Build history of the part. All positions in model axes, mm. A direction names the side the tool comes from. Coordinates: 2 decimals unless noted, no trailing zeros. Order: outer loops, then holes, each group sorted by start corner. A loop starts at its lowest first (then second) coordinate and runs counter-clockwise, first axis right, second up. Notation, with made-up numbers: (8.5, -10.75) - (13.5, -10.75) arc R14 ccw to (13.5, 10.25) - close; hole circle Ø2 at (-37, 20.25). An arc over 180 degrees is marked (long way). Answer as CSV lines item,"result". Start each with the question number.
from build123d import *

# Parameters (mm, degrees)
BOSS_EXTRUDE1_DEPTH = 90
SKETCH2_R           = 2
CUT_EXTRUDE1_DEPTH  = 26
BOSS_EXTRUDE2_DEPTH = 90
SKETCH4_W           = 47.922407602
SKETCH4_H           = 26.699627092
BOSS_EXTRUDE3_DEPTH = 20
SKETCH7_R           = 2.5
CUT_EXTRUDE2_DEPTH  = 66.5
SKETCH9_W           = 15
SKETCH9_H           = 8
CUT_EXTRUDE3_DEPTH  = 91
CUT_EXTRUDE4_REACH  = 62.6
SKETCH8_R           = 2.5
CUT_EXTRUDE5_DEPTH  = 67
SKETCH12_W          = 63.84660413
SKETCH12_H          = 90
BOSS_EXTRUDE4_DEPTH = 67
BOSS_EXTRUDE5_START = -3
SKETCH13_R          = 10
BOSS_EXTRUDE5_DEPTH = 31
SKETCH15_R          = 12.5
BOSS_EXTRUDE6_DEPTH = 3
SKETCH16_R          = 12.5
BOSS_EXTRUDE7_DEPTH = 3
SKETCH17_W          = 34
SKETCH17_H          = 34
CUT_EXTRUDE6_DEPTH  = 2
SKETCH18_R          = 10
CUT_EXTRUDE7_DEPTH  = 5
SKETCH19_R          = 12.5
CUT_EXTRUDE8_DEPTH  = 3


with BuildPart() as part:
    # Sketch1 → Boss-Extrude1 (new body)
    with BuildSketch(Plane.XY):
        Polygon((-283, 0), (0, 0), (0, 15), (-217.53, 15), (-217.53, 11), (-237.53, 11), (-237.53, 15), (-254.5, 15), (-254.5, 11), (-274, 11), (-274, 15), (-283, 15), align=None)
    extrude(amount=BOSS_EXTRUDE1_DEPTH)

    # Sketch2 → Cut-Extrude1 (cut)
    with BuildSketch(Plane(origin=(0, 15, 0), x_dir=(1, 0, 0), z_dir=(0, 1, 0))):
        with Locations((-246.015, -45)):
            Circle(SKETCH2_R)
    extrude(amount=-CUT_EXTRUDE1_DEPTH, mode=Mode.SUBTRACT)

    # Sketch3 → Boss-Extrude2 (add)
    with BuildSketch(Plane(origin=(0, 0, 0), x_dir=(-1, 0, 0), z_dir=(0, 0, -1))):
        Polygon((0, 0), (0, -61.6), (0, -69.046795722), (8.076697935, -69.046795722), (16.610633667, -45.6), (63.389366333, -45.6), (71.923302065, -69.046795722), (128.076697935, -69.046795722), (136.610633667, -45.6), (183.389366333, -45.6), (191.923302065, -69.046795722), (200, -69.046795722), (200, -61.6), (200, 7.5), (0, 7.5), align=None)
    extrude(amount=-BOSS_EXTRUDE2_DEPTH)

    # Sketch4 → Boss-Extrude3 (add, symmetric)
    with BuildSketch(Plane(origin=(0, 0, 44.5), x_dir=(-1, 0, 0), z_dir=(0, 0, -1))):
        with Locations((40.197751444, -51.696982176)):
            Rectangle(SKETCH4_W, SKETCH4_H)
    extrude(amount=BOSS_EXTRUDE3_DEPTH, both=True)

    # Sketch7 → Cut-Extrude2 (cut, through all)
    with BuildSketch(Plane(origin=(0, 0, 24.5), x_dir=(-1, 0, 0), z_dir=(0, 0, -1))):
        with Locations((40, -61.6)):
            Circle(SKETCH7_R)
    extrude(amount=-CUT_EXTRUDE2_DEPTH, mode=Mode.SUBTRACT)

    # Sketch9 → Cut-Extrude3 (cut, through all)
    with BuildSketch(Plane(origin=(0, 0, 0), x_dir=(-1, 0, 0), z_dir=(0, 0, -1))):
        with Locations((160, -36.6)):
            Rectangle(SKETCH9_W, SKETCH9_H)
    extrude(amount=-CUT_EXTRUDE3_DEPTH, mode=Mode.SUBTRACT)

    # Sketch8 → Cut-Extrude4 (cut, up to next)
    with BuildSketch(Plane.XZ.offset(45.6), mode=Mode.PRIVATE) as cut_extrude4_sk1:
        with Locations((-160, 75)):
            Circle(SKETCH8_R)
    cut_extrude4_tool1 = extrude(cut_extrude4_sk1.sketch, amount=-CUT_EXTRUDE4_REACH, mode=Mode.PRIVATE) & part.part
    add(cut_extrude4_tool1.solids().sort_by_distance((-160, -45.6, 75))[0], mode=Mode.SUBTRACT)
    # Sketch8 → Cut-Extrude4 (cut, up to next)
    with BuildSketch(Plane.XZ.offset(45.6), mode=Mode.PRIVATE) as cut_extrude4_sk2:
        with Locations((-160, 15)):
            Circle(SKETCH8_R)
    cut_extrude4_tool2 = extrude(cut_extrude4_sk2.sketch, amount=-CUT_EXTRUDE4_REACH, mode=Mode.PRIVATE) & part.part
    add(cut_extrude4_tool2.solids().sort_by_distance((-160, -45.6, 15))[0], mode=Mode.SUBTRACT)

    # Sketch10 → Cut-Extrude5 (cut)
    with BuildSketch(Plane.XZ.offset(69.046795722)):
        Polygon((-8.076697935, 90), (-90, 90), (-90, 0), (-8.076697935, 0), (0, 0), (0, 90), align=None)
    extrude(amount=-CUT_EXTRUDE5_DEPTH, mode=Mode.SUBTRACT)

    # Sketch12 → Boss-Extrude4 (add)
    with BuildSketch(Plane.XZ.offset(69.046795722)):
        with Locations((-160, 45)):
            Rectangle(SKETCH12_W, SKETCH12_H)
    extrude(amount=-BOSS_EXTRUDE4_DEPTH)

    # Sketch13 → Boss-Extrude5 (add)
    with BuildSketch(Plane.XY.offset(90).offset(BOSS_EXTRUDE5_START)):
        with Locations((-175, -41.946795722)):
            Circle(SKETCH13_R)
    boss_extrude5 = extrude(amount=BOSS_EXTRUDE5_DEPTH)

    # Sketch15 → Boss-Extrude6 (add)
    with BuildSketch(Plane.XY.offset(118)):
        with Locations((-175, -41.946795722)):
            Circle(SKETCH15_R)
    boss_extrude6 = extrude(amount=-BOSS_EXTRUDE6_DEPTH)

    # Mirror1: Boss-Extrude5, Boss-Extrude6 across plane
    add(boss_extrude5.mirror(Plane(origin=(0, 0, 44.5), x_dir=(1, 0, 0), z_dir=(0, 0, -1))))
    add(boss_extrude6.mirror(Plane(origin=(0, 0, 44.5), x_dir=(1, 0, 0), z_dir=(0, 0, -1))))

    # Sketch16 → Boss-Extrude7 (add)
    with BuildSketch(Plane.XY.offset(90)):
        with Locations((-175, -41.946795722)):
            Circle(SKETCH16_R)
    boss_extrude7 = extrude(amount=BOSS_EXTRUDE7_DEPTH)

    # Mirror2: Boss-Extrude7 across plane
    add(boss_extrude7.mirror(Plane(origin=(0, 0, 44.5), x_dir=(1, 0, 0), z_dir=(0, 0, -1))))

    # Sketch17 → Cut-Extrude6 (cut)
    with BuildSketch(Plane(origin=(0, -2.046795722, 0), x_dir=(-1, 0, 0), z_dir=(0, -1, 0))):
        with Locations((37, -45)):
            Rectangle(SKETCH17_W, SKETCH17_H)
    extrude(amount=-CUT_EXTRUDE6_DEPTH, mode=Mode.SUBTRACT)

    # Sketch18 → Cut-Extrude7 (cut)
    with BuildSketch(Plane.XZ.offset(0.046795722)):
        with Locations((-37, 45)):
            Circle(SKETCH18_R)
    extrude(amount=-CUT_EXTRUDE7_DEPTH, mode=Mode.SUBTRACT)

    # Sketch19 → Cut-Extrude8 (cut)
    with BuildSketch(Plane.XZ.offset(-4.953204278)):
        with Locations((-37, 45)):
            Circle(SKETCH19_R)
    extrude(amount=-CUT_EXTRUDE8_DEPTH, mode=Mode.SUBTRACT)


solid = part.part
(1) Band-saw the part on A-A on z = 77. List the corners of the cut face in (x, y), plus the area to 3 significant figures.
(2) Band-saw the part on D-D on x = -79. List the corners of the cut face in (y, z), plus the area to 3 significant figures.
(3) Pull direction Z, two halves, no side cores. Call faces 6 (the flat face through (-90, -36, 46)), 7 (the cylindrical face through (-165.763, -45.777, 103.846)), 8 (the flat face through (-175, -42, 118)): +Z half, -Z half, draft (parallel to the pull), parting line (faces both ways), or undercut.
(4) Drop flat-ended pins along their axis: pin 1 Ø6 at (x, z) = (-265.5, 63.5) entering from +Y; pin 2 Ø0.6 at (y, z) = (-0.5, 50.5) entering from -X; pin 3 Ø12 at (x, y) = (-199.5, -52.5) entering from +Z. Give the stop position or say it passes through.
(5) Probe L1, parallel to Z at x = -37, y = 1.1; L2, parallel to Z at x = -37, y = 6.1; L3, parallel to X at y = 8, z = 45 (3 decimals). List the from-to ranges inside material, lowest first. Write a range as [from, to].
(6) Which spindle directions (+Z, -Z, +X, -X, +Y, -Y) get a long thin tool onto all of the face, cutting with end or side? Do faces 1 (the cylindrical face through (-163.077, -38.192, 116.521)), 2 (the flat face through (-227, 11, 44)), 3 (the flat face through (-44.3, -0.047, 52.3)), 4 (the cylindrical face through (-163.077, -38.192, -27.521)), 5 (the flat face through (-175.1, -31.7, 115)). Say none if no direction does.
Filled in:
1,outline,"(-283, 0) - (-200, 0) - (-200, -69.05) - (-90, -69.05) - (-90, -2.05) - (0, -2.05) - (0, 15) - (-217.53, 15) - (-217.53, 11) - (-237.53, 11) - (-237.53, 15) - (-254.5, 15) - (-254.5, 11) - (-274, 11) - (-274, 15) - (-283, 15) - close"
1,area,"11,900 mm^2"
2,outline,"(-2.05, 0) - (15, 0) - (15, 90) - (-2.05, 90) - close"
2,area,"1,530 mm^2"
3,face 6,"draft"
3,face 7,"undercut"
3,face 8,"+Z half"
4,pin 1,"stops at y = 11"
4,pin 2,"stops at x = -200"
4,pin 3,"stops at z = 90"
5,L1,"z = [0, 35], [55, 90]"
5,L2,"z = [0, 32.5], [57.5, 90]"
5,L3,"x = [-283, -248.015], [-244.015, 0]"
6,face 1,"+Z"
6,face 2,"+Z, -Z, +Y"
6,face 3,"-Y"
6,face 4,"-Z"
6,face 5,"none"
